from build123d import *

# Parameters (mm, degrees)
BOSS_EXTRU_1_DEPTH        = 27.175
BOSS_EXTRU_1_DEPTH_BACK   = 3.175
BOSS_EXTRU_1_2_DEPTH      = 27.175
BOSS_EXTRU_1_2_DEPTH_BACK = 3.175
BOSS_EXTRU_1_3_DEPTH      = 27.175
BOSS_EXTRU_1_3_DEPTH_BACK = 3.175
BOSS_EXTRU_1_4_DEPTH      = 27.175
BOSS_EXTRU_1_4_DEPTH_BACK = 3.175
BOSS_EXTRU_1_5_DEPTH      = 27.175
BOSS_EXTRU_1_5_DEPTH_BACK = 3.175
BOSS_EXTRU_1_6_DEPTH      = 27.175
BOSS_EXTRU_1_6_DEPTH_BACK = 3.175
BOSS_EXTRU_1_7_DEPTH      = 27.175
BOSS_EXTRU_1_7_DEPTH_BACK = 3.175
BOSS_EXTRU_2_DEPTH        = 198.346
BOSS_EXTRU_2_DEPTH_BACK   = 218.854
ESQUISSE2_W               = 3.175
ESQUISSE2_H               = 24


with BuildPart() as part:
    # Esquisse1 → Boss.-Extru.1 (new, two sides: drawn at the far end of the back side and taken through both)
    with BuildSketch(Plane.XY.offset(-BOSS_EXTRU_1_DEPTH_BACK)):
        Polygon((-43, 163.6), (-43, 163.346), (-39.825, 163.346), (-39.825, 163.6), (-39.825, 183.6), (-39.825, 183.854), (-43, 183.854), (-43, 183.6), align=None)
    extrude(amount=BOSS_EXTRU_1_DEPTH + BOSS_EXTRU_1_DEPTH_BACK)



with BuildPart() as body_2:
    # Esquisse1 → Boss.-Extru.1 2 (new, two sides: drawn at the far end of the back side and taken through both)
    with BuildSketch(Plane.XY.offset(-BOSS_EXTRU_1_2_DEPTH_BACK)):
        Polygon((-43, 125.733333333), (-43, 125.987333333), (-39.825, 125.987333333), (-39.825, 125.733333333), (-39.825, 105.733333333), (-39.825, 105.479333333), (-43, 105.479333333), (-43, 105.733333333), align=None)
    extrude(amount=BOSS_EXTRU_1_2_DEPTH + BOSS_EXTRU_1_2_DEPTH_BACK)


with BuildPart() as body_3:
    # Esquisse1 → Boss.-Extru.1 3 (new, two sides: drawn at the far end of the back side and taken through both)
    with BuildSketch(Plane.XY.offset(-BOSS_EXTRU_1_3_DEPTH_BACK)):
        Polygon((-43, 67.866666667), (-43, 68.120666667), (-39.825, 68.120666667), (-39.825, 67.866666667), (-39.825, 47.866666667), (-39.825, 47.612666667), (-43, 47.612666667), (-43, 47.866666667), align=None)
    extrude(amount=BOSS_EXTRU_1_3_DEPTH + BOSS_EXTRU_1_3_DEPTH_BACK)


with BuildPart() as body_4:
    # Esquisse1 → Boss.-Extru.1 4 (new, two sides: drawn at the far end of the back side and taken through both)
    with BuildSketch(Plane.XY.offset(-BOSS_EXTRU_1_4_DEPTH_BACK)):
        Polygon((-43, 10), (-43, 10.254), (-39.825, 10.254), (-39.825, 10), (-39.825, -10), (-39.825, -10.254), (-43, -10.254), (-43, -10), align=None)
    extrude(amount=BOSS_EXTRU_1_4_DEPTH + BOSS_EXTRU_1_4_DEPTH_BACK)


with BuildPart() as body_5:
    # Esquisse1 → Boss.-Extru.1 5 (new, two sides: drawn at the far end of the back side and taken through both)
    with BuildSketch(Plane.XY.offset(-BOSS_EXTRU_1_5_DEPTH_BACK)):
        Polygon((-43, -163.6), (-43, -183.6), (-43, -183.854), (-39.825, -183.854), (-39.825, -183.6), (-39.825, -163.6), (-39.825, -163.346), (-43, -163.346), align=None)
    extrude(amount=BOSS_EXTRU_1_5_DEPTH + BOSS_EXTRU_1_5_DEPTH_BACK)


with BuildPart() as body_6:
    # Esquisse1 → Boss.-Extru.1 6 (new, two sides: drawn at the far end of the back side and taken through both)
    with BuildSketch(Plane.XY.offset(-BOSS_EXTRU_1_6_DEPTH_BACK)):
        Polygon((-43, -105.733333333), (-43, -125.733333333), (-43, -125.987333333), (-39.825, -125.987333333), (-39.825, -125.733333333), (-39.825, -105.733333333), (-39.825, -105.479333333), (-43, -105.479333333), align=None)
    extrude(amount=BOSS_EXTRU_1_6_DEPTH + BOSS_EXTRU_1_6_DEPTH_BACK)


with BuildPart() as body_7:
    # Esquisse1 → Boss.-Extru.1 7 (new, two sides: drawn at the far end of the back side and taken through both)
    with BuildSketch(Plane.XY.offset(-BOSS_EXTRU_1_7_DEPTH_BACK)):
        Polygon((-43, -47.866666667), (-43, -67.866666667), (-43, -68.120666667), (-39.825, -68.120666667), (-39.825, -67.866666667), (-39.825, -47.866666667), (-39.825, -47.612666667), (-43, -47.612666667), align=None)
    extrude(amount=BOSS_EXTRU_1_7_DEPTH + BOSS_EXTRU_1_7_DEPTH_BACK)


with BuildPart() as part_1:
    add(part.part)

    add(body_2.part)  # Boss.-Extru.2 merges body 2

    add(body_3.part)  # Boss.-Extru.2 merges body 3

    add(body_4.part)  # Boss.-Extru.2 merges body 4

    add(body_5.part)  # Boss.-Extru.2 merges body 5

    add(body_6.part)  # Boss.-Extru.2 merges body 6

    add(body_7.part)  # Boss.-Extru.2 merges body 7
    # Esquisse2 → Boss.-Extru.2 (add, two sides: drawn at the far end of the back side and taken through both)
    with BuildSketch(Plane.XZ.offset(10.254).offset(-BOSS_EXTRU_2_DEPTH_BACK)):
        with Locations((-41.4125, 12)):
            Rectangle(ESQUISSE2_W, ESQUISSE2_H)
    extrude(amount=BOSS_EXTRU_2_DEPTH + BOSS_EXTRU_2_DEPTH_BACK)


solid = part_1.part
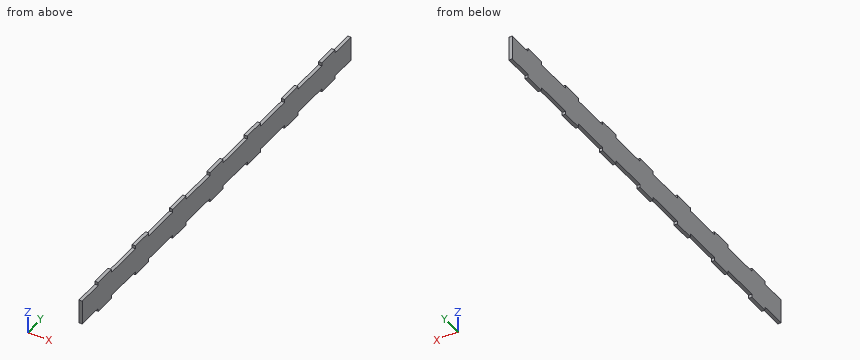
Check sheet for the modelled part. Datum: model origin and axes. Units: mm. Round coordinates to 2 decimals unless told otherwise and drop trailing zeros. Order: outer loops, then holes, each group sorted by start corner. A loop starts at its lowest first (then second) coordinate and runs counter-clockwise, first axis right, second up. Notation, with made-up numbers: M -25,-34.5 L 17,-34.5 A24 cw 17,-1.5 Z; hole C 1.5,-20.75 d11. An arc over 180 degrees is marked long. One line per item, written item: value. Start each with the question number.
1. Section check A-A on y = -101. Enter the section's corners in (x, z) (3 decimals), and give its area (3 significant figures).
2. Gauge pin test, flat ends, axial feed: P1, Ø1, axis at x = -41, y = -194, coming from the -Z side; P2, Ø1.6, axis at x = -41.5, z = -1.5, coming from the +Y side; P3, Ø1.6, axis at x = -41, z = -1.5, coming from the -Y side. Record the tip position at first contact, or that the pin passes through.
3. Scan line: line 1 along Z through (x, y) = (-42.1, 131). Record every from-to range of solid material in increasing order.
Results found:
1. outline: M -43,0 L -39.825,0 L -39.825,24 L -43,24 Z
1. area: 76.2 mm^2
2. P1: z = 0
2. P2: y = 183.85
2. P3: y = -183.85
3. line 1: 0 to 24
